Can you work these out from the model? Positions are in its coordinate system, mm. A direction names the side the tool comes from. Round coordinates to 2 decimals unless told otherwise and drop trailing zeros. Loops run counter-clockwise (first coordinate to the right, second up) from the corner with the lowest first, then second, coordinate; pieces in that order, holes last. Notation, with made-up numbers: M 7,-26 L 46,-26 A28 cw 46,-4 Z; hole C 72,62 d11. An arc over 180 degrees is marked long. Answer as CSV lines item,"result".
from build123d import *

# Parameters (mm, degrees)
F1_DEPTH = 25
F2_ANGLE = 30
F4_DEPTH = 25
F6_START = 7.5
F6_DEPTH = 10


with BuildPart() as f1:
    # F0 (on Front) → F1 (new body)
    with BuildSketch(Plane.XZ):
        Polygon((59.6599376417, 0), (59.6599376417, 10), (-0.3400623583, 10), (-0.3400623583, 31.4), (59.6599376417, 31.4), (59.6599376417, 41.4), (-10.3400623583, 41.4), (-10.3400623583, 0), align=None)
    extrude(amount=F1_DEPTH)


with BuildPart() as f1_1:
    # F2: moved
    add(f1.part.rotate(Axis((-10.3400623583, -12.5, 0), (0, 1, 0)), F2_ANGLE))

    # F3 (on Front) → F4 (join)
    with BuildSketch(Plane.XZ):
        Polygon((36.3406997552, 20.8534517167), (62.3214618687, 5.8534517167), (262.3214618687, 352.2636132305), (236.3406997552, 367.2636132305), align=None)
    extrude(amount=F4_DEPTH)

    # F5 (on Front) → F6 (join)
    with BuildSketch(Plane.XZ.offset(F6_START)):
        Polygon((23.3896902468, 28.3307205427), (31.9308649473, 43.1244690803), (23.0304820152, 48.263107562), (14.4893073146, 33.4693590244), align=None)
    extrude(amount=F6_DEPTH)


solid = f1_1.part
Item 1: If we section it at A-A on z = 11.5: Write out the boundary of the cut face in (x, y), then the cut area to 3 significant figures.
Output:
outline,"M -3.7,-25 L 7.85,-25 L 7.85,0 L -3.7,0 Z; M 32.54,-25 L 65.58,-25 L 65.58,0 L 32.54,0 Z"
area,"1,110 mm2"
Item 2: If we section it at B-B on x = 220: Write out the boundary of the cut face in (y, z).
Output:
outline,"M -25,278.96 L 0,278.96 L 0,338.96 L -25,338.96 Z"
Item 3: Will these pins go through, and if not, where does the flat tip stop? pin 1 (3 mm diameter, centred on y = -5.5, z = 205, fed in from +X); pin 2 (10 mm diameter, centred on x = 31, y = -12.5, fed in from -Z); pin 3 (14 mm diameter, centred on x = 20, z = 42, fed in from -Y).
Output:
pin 1,"stops at x = 178.16"
pin 2,"stops at z = -26.75"
pin 3,"stops at y = -17.5"
Item 4: We'd pull the mould along Z, two halves only. Please class faces 6 (the face through (23, -7.5, 38)), 7 (the face through (27.54, -12.43, 45.66)), 8 (the face through (66.71, -12.32, 3.32)): released by +Z, released by -Z, zero draft, split by the parting line, or undercut.
Output:
face 6,"zero draft"
face 7,"released by +Z"
face 8,"undercut"
Item 5: If we section it at C-C on z = 124.5: Write out the boundary of the cut face in (x, y).
Output:
outline,"M 96.18,-25 L 130.82,-25 L 130.82,0 L 96.18,0 Z"
Item 6: On a 3-axis mill with a long thin cutter (end or side, diameter ignored), from which of +Z, -Z, +X, -X, +Y, -Y can I reach the whole of each face in a straight line? I mean faces 1 (the face through (23.53, -12.32, 28.25)), 2 (the face through (138, 0, 173)), 3 (the face through (0.155, -12.325, 18.178)), 4 (the face through (23, -17.5, 38)), 5 (the face through (39.64, -12.32, 7.4)). Say none if no direction works.
Output:
face 1,"none"
face 2,"+Z, -Z, +X, -X, +Y"
face 3,"+Z, -X, +Y, -Y"
face 4,"+Z, -Y"
face 5,"+Y, -Y"
Item 7: If I drill on line 1 along X through (y, z) = (-10, 22); line 2 along X through (y, z) = (-1, 21.5) (3 decimals); line 3 along Z through (x, y) = (66, -15.75), over which ranges is the centre line in solid material (lowest first)? Write a range as from..to.
Output:
line 1,"x = 2.36..13.91, 14.35..34.35, 37..71.64"
line 2,"x = 2.073..13.62, 15.221..35.221, 36.714..71.355"
line 3,"z = -7.78..3.73, 12.22..72.22"
